Could you check a few things on this drawing? It's one solid part, dimensions in mm from its lowest x, y, z. A direction names the side the tool comes from. Give positions to 0.01 mm unless a question says otherwise; leave off trailing zeros. Order: outer loops, then holes, each group sorted by start corner. A loop starts at its lowest first (then second) coordinate and runs counter-clockwise, first axis right, second up. Notation, with made-up numbers: (45.5, 21.25) - (51.5, 21.25) arc R19 cw to (51.5, 45.25) - close; hole circle Ø10 at (72, 80.5). An arc over 180 degrees is marked (long way). One line per question, with ' | ' between items. Start each with the question number.
1. For P1, Ø1.5, axis at x = 48.5, z = 13, coming from the +Y side; P2, Ø8.5, axis at x = 40, z = 41, coming from the +Y side; P3, Ø7.5, axis at y = 40, z = 41, coming from the -X side; P4, Ø8, axis at x = 29.5, y = 61, coming from the -Z side, each with a flat end and sliding along its axis, tell me the tip position at first contact or that it passes through.
2. Imagine slicing it at C-C (z = 18). Please give me the cut outline in (x, y), and give its area (3 significant figures).
3. Which directions (+Z, -Z, +X, -X, +Y, -Y) give clear straight access to the entire face, cutting with the end or side of a thin tool? Please do the marked faces 4, 5 and 6.
4. Imagine slicing it at A-A (x = 40). Give the number of separate pieces and of enclosed holes in the cut face, and give its area (3 significant figures).
5. If we mould it in two halves opening along Z, with no side actions, what happens to the marked faces 1, 2 and 3? For each: released by +Z, released by -Z, zero draft, split by the parting line, or undercut.
6. I need wall thicknesses on probe 1 along Y at (x, z) = (40, 28.5); probe 2 along Z at (x, y) = (40, 63.75); probe 3 along Z at (x, y) = (67, 45.5). Which ranges of each line are inside material? Lowest first, please. Write a range as from..to.
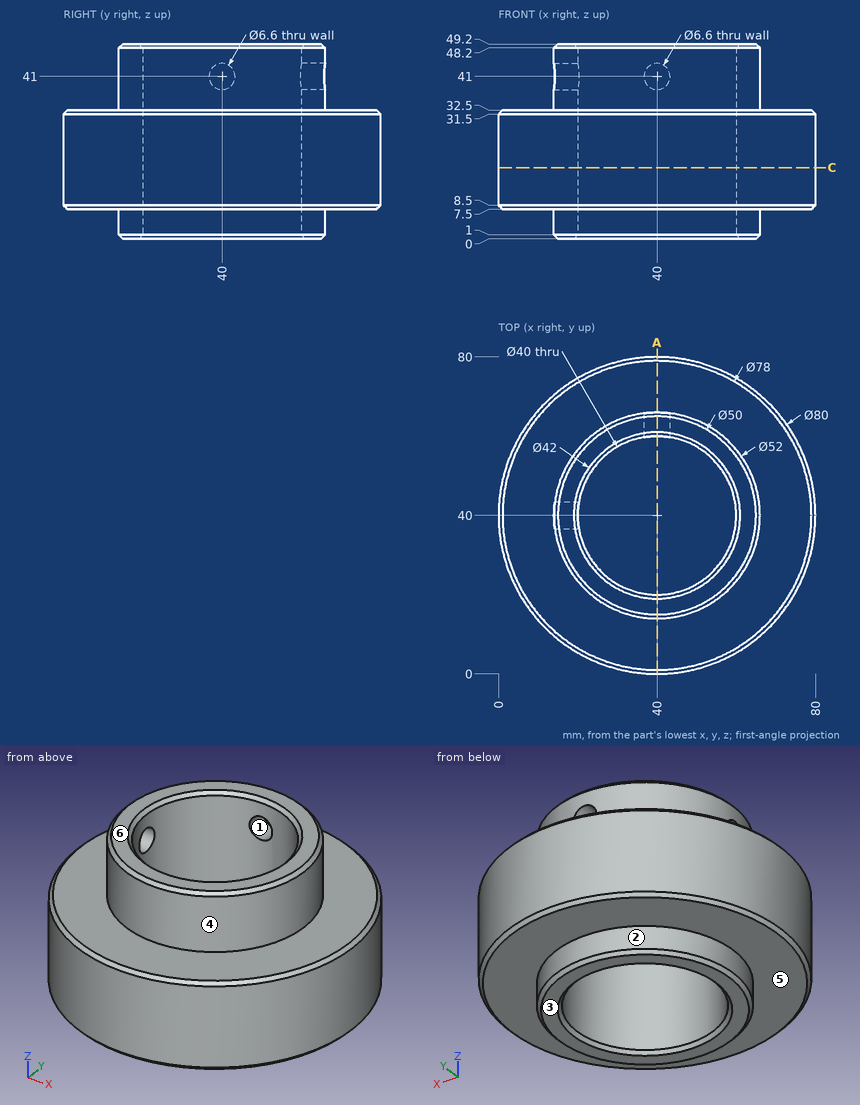
Results found:
1) P1: stops at y = 79.24 | P2: stops at y = 66 | P3: stops at x = 14 | P4: stops at z = 0
2) outline: circle Ø80 at (40, 40); hole circle Ø40 at (40, 40) | area: 3,770 mm2
3) face 4: +Z | face 5: -Z | face 6: +Z, +X, -X, +Y, -Y
4) separate pieces: 3 | enclosed holes: 0 | area: 1,240 mm2
5) face 1: undercut | face 2: zero draft | face 3: released by -Z
6) probe 1: y = 0..20, 60..80 | probe 2: z = 0..37.7, 44.3..49.2 | probe 3: z = 7.5..32.5
